Can you work these out from the model? Positions are in its coordinate system, mm. A direction names the side the tool comes from. Give positions to 0.01 mm unless a question says otherwise; leave off trailing zeros. Order: outer loops, then holes, each group sorted by start corner. A loop starts at its lowest first (then second) coordinate and runs counter-clockwise, first axis right, second up. Notation, with made-up numbers: (5.5, -32.5) -> (28.5, -32.5) arc R35 cw to (28.5, 3.5) -> close; hole circle Ø2 at (-11, 48). An arc over 180 degrees is marked (long way). Answer as CSV lines item,"result".
```python
from build123d import *

# Parameters (mm, degrees)
SKETCH1_R           = 2.1
BOSS_EXTRUDE1_DEPTH = 90
SKETCH5_R           = 2.5
CUT_EXTRUDE1_DEPTH  = 5
SKETCH6_R           = 8.4
SKETCH6_R_2         = 8
CUT_EXTRUDE2_DEPTH  = 4.2
FILLET1_START       = -1
FILLET1_DEPTH       = 5.2
CUT_EXTRUDE3_START  = -8
SKETCH7_R           = 8.4
SKETCH7_R_2         = 8
CUT_EXTRUDE3_DEPTH  = 8
SKETCH8_R           = 4.3
CUT_EXTRUDE4_DEPTH  = 4.2
FILLET2_START       = 82
FILLET2_DEPTH       = 9
SKETCH9_R           = 5
CUT_EXTRUDE5_DEPTH  = 85.8
SKETCH10_R          = 4.2
CUT_EXTRUDE6_DEPTH  = 4.2
BOSS_EXTRUDE2_START = 1.4
SKETCH11_W          = 90
SKETCH11_H          = 20
SKETCH11_R          = 2.5
BOSS_EXTRUDE2_DEPTH = 1.4


with BuildPart() as part:
    # Sketch1 → Boss-Extrude1 (new body)
    with BuildSketch(Plane.XY):
        with BuildLine():
            Line((8.4, 0), (31.8, 0))
            ThreePointArc((31.8, 0), (37.739696962, 2.460303038), (40.2, 8.4))
            Line((40.2, 8.4), (40.2, 31.8))
            ThreePointArc((40.2, 31.8), (37.739696962, 37.739696962), (31.8, 40.2))
            Line((31.8, 40.2), (8.4, 40.2))
            ThreePointArc((8.4, 40.2), (2.460303038, 37.739696962), (0, 31.8))
            Line((0, 31.8), (0, 8.4))
            ThreePointArc((0, 8.4), (2.460303038, 2.460303038), (8.4, 0))
        make_face()
        with Locations(Location((8.4, 31.8, 0), (0, 0, 180))):
            Circle(SKETCH1_R, mode=Mode.SUBTRACT)
        with Locations(Location((31.8, 31.8, 0), (0, 0, 180))):
            Circle(SKETCH1_R, mode=Mode.SUBTRACT)
        with Locations(Location((31.8, 8.4, 0), (0, 0, 180))):
            Circle(SKETCH1_R, mode=Mode.SUBTRACT)
        with Locations(Location((8.4, 8.4, 0), (0, 0, 180))):
            Circle(SKETCH1_R, mode=Mode.SUBTRACT)
    extrude(amount=BOSS_EXTRUDE1_DEPTH)

    # Sketch5 → Cut-Extrude1 (cut)
    with BuildSketch(Plane(origin=(40.2, 0, 0), x_dir=(0, 0, -1), z_dir=(1, 0, 0))):
        with Locations((-82, 20.1)):
            Circle(SKETCH5_R)
        with Locations((-8, 20.1)):
            Circle(SKETCH5_R)
    extrude(amount=-CUT_EXTRUDE1_DEPTH, mode=Mode.SUBTRACT)

    # Sketch6 → Cut-Extrude2 (cut)
    # profile 1 of 4: a face of its own
    with BuildSketch(Plane(origin=(0, 0, 0), x_dir=(-1, 0, 0), z_dir=(0, 0, -1))):
        with Locations((-31.8, 31.8)):
            Circle(SKETCH6_R)
        with Locations((-31.8, 31.8)):
            Circle(SKETCH6_R_2, mode=Mode.SUBTRACT)
    # profile 2 of 4: a face of its own
    with BuildSketch(Plane(origin=(0, 0, 0), x_dir=(-1, 0, 0), z_dir=(0, 0, -1))):
        with Locations((-8.4, 31.8)):
            Circle(SKETCH6_R)
        with Locations((-8.4, 31.8)):
            Circle(SKETCH6_R_2, mode=Mode.SUBTRACT)
    # profile 3 of 4: a face of its own
    with BuildSketch(Plane(origin=(0, 0, 0), x_dir=(-1, 0, 0), z_dir=(0, 0, -1))):
        with Locations((-8.4, 8.4)):
            Circle(SKETCH6_R)
        with Locations((-8.4, 8.4)):
            Circle(SKETCH6_R_2, mode=Mode.SUBTRACT)
    # profile 4 of 4: a face of its own
    with BuildSketch(Plane(origin=(0, 0, 0), x_dir=(-1, 0, 0), z_dir=(0, 0, -1))):
        with Locations((-31.8, 8.4)):
            Circle(SKETCH6_R)
        with Locations((-31.8, 8.4)):
            Circle(SKETCH6_R_2, mode=Mode.SUBTRACT)
    extrude(amount=-CUT_EXTRUDE2_DEPTH, mode=Mode.SUBTRACT)

    # Fillet1: read off the stored shape, not the designer's step
    # Fillet1 outline → Fillet1 (cut)
    with BuildSketch(Plane.XY.offset(FILLET1_START)):
        with BuildLine():
            ThreePointArc((0, 8.4), (0.024888944, 9.046153846), (0.099408284, 9.688478624))
            ThreePointArc((0.099408284, 9.688478624), (0.046153846, 9.646296288), (0, 9.69614814))
            Line((0, 9.69614814), (0, 8.4))
        make_face()
        with BuildLine():
            ThreePointArc((9.69614814, 0), (9.646296288, 0.046153846), (9.688478624, 0.099408284))
            ThreePointArc((9.688478624, 0.099408284), (9.046153846, 0.024888944), (8.4, 0))
            Line((8.4, 0), (9.69614814, 0))
        make_face()
        with BuildLine():
            Line((0, 31.8), (0, 30.50385186))
            ThreePointArc((0, 30.50385186), (0.046153846, 30.553703712), (0.099408284, 30.511521376))
            ThreePointArc((0.099408284, 30.511521376), (0.024888944, 31.153846154), (0, 31.8))
        make_face()
        with BuildLine():
            ThreePointArc((30.511521376, 0.099408284), (30.553703712, 0.046153846), (30.50385186, 0))
            Line((30.50385186, 0), (31.8, 0))
            ThreePointArc((31.8, 0), (31.153846154, 0.024888944), (30.511521376, 0.099408284))
        make_face()
        with BuildLine():
            ThreePointArc((8.4, 40.2), (9.046153846, 40.175111056), (9.688478624, 40.100591716))
            ThreePointArc((9.688478624, 40.100591716), (9.646296288, 40.153846154), (9.69614814, 40.2))
            Line((9.69614814, 40.2), (8.4, 40.2))
        make_face()
        with BuildLine():
            ThreePointArc((40.2, 9.69614814), (40.153846154, 9.646296288), (40.100591716, 9.688478624))
            ThreePointArc((40.100591716, 9.688478624), (40.175111056, 9.046153846), (40.2, 8.4))
            Line((40.2, 8.4), (40.2, 9.69614814))
        make_face()
        with BuildLine():
            Line((31.8, 40.2), (30.50385186, 40.2))
            ThreePointArc((30.50385186, 40.2), (30.553703712, 40.153846154), (30.511521376, 40.100591716))
            ThreePointArc((30.511521376, 40.100591716), (31.153846154, 40.175111056), (31.8, 40.2))
        make_face()
        with BuildLine():
            ThreePointArc((40.100591716, 30.511521376), (40.153846154, 30.553703712), (40.2, 30.50385186))
            Line((40.2, 30.50385186), (40.2, 31.8))
            ThreePointArc((40.2, 31.8), (40.175111056, 31.153846154), (40.100591716, 30.511521376))
        make_face()
    extrude(amount=FILLET1_DEPTH, mode=Mode.SUBTRACT)

    # Sketch7 → Cut-Extrude3 (cut)
    # profile 1 of 4: a face of its own
    with BuildSketch(Plane.XY.offset(90).offset(CUT_EXTRUDE3_START)):
        with Locations((8.4, 31.8)):
            Circle(SKETCH7_R)
        with Locations(Location((8.4, 31.8, 0), (0, 0, 180))):
            Circle(SKETCH7_R_2, mode=Mode.SUBTRACT)
    # profile 2 of 4: a face of its own
    with BuildSketch(Plane.XY.offset(90).offset(CUT_EXTRUDE3_START)):
        with Locations((31.8, 31.8)):
            Circle(SKETCH7_R)
        with Locations(Location((31.8, 31.8, 0), (0, 0, 180))):
            Circle(SKETCH7_R_2, mode=Mode.SUBTRACT)
    # profile 3 of 4: a face of its own
    with BuildSketch(Plane.XY.offset(90).offset(CUT_EXTRUDE3_START)):
        with Locations((31.8, 8.4)):
            Circle(SKETCH7_R)
        with Locations(Location((31.8, 8.4, 0), (0, 0, 180))):
            Circle(SKETCH7_R_2, mode=Mode.SUBTRACT)
    # profile 4 of 4: a face of its own
    with BuildSketch(Plane.XY.offset(90).offset(CUT_EXTRUDE3_START)):
        with Locations((8.4, 8.4)):
            Circle(SKETCH7_R)
        with Locations(Location((8.4, 8.4, 0), (0, 0, 180))):
            Circle(SKETCH7_R_2, mode=Mode.SUBTRACT)
    extrude(amount=CUT_EXTRUDE3_DEPTH, mode=Mode.SUBTRACT)

    # Sketch8 → Cut-Extrude4 (cut)
    with BuildSketch(Plane.XY.offset(90)):
        with Locations((8.4, 31.8)):
            Circle(SKETCH8_R)
        with Locations((31.8, 31.8)):
            Circle(SKETCH8_R)
        with Locations((31.8, 8.4)):
            Circle(SKETCH8_R)
        with Locations((8.4, 8.4)):
            Circle(SKETCH8_R)
    extrude(amount=-CUT_EXTRUDE4_DEPTH, mode=Mode.SUBTRACT)

    # Fillet2: read off the stored shape, not the designer's step
    # Fillet2 outline → Fillet2 (cut)
    with BuildSketch(Plane.XY.offset(FILLET2_START)):
        with BuildLine():
            ThreePointArc((0.099408284, 9.688478624), (0.046153846, 9.646296288), (0, 9.69614814))
            Line((0, 9.69614814), (0, 8.4))
            ThreePointArc((0, 8.4), (0.024888944, 9.046153846), (0.099408284, 9.688478624))
        make_face()
        with BuildLine():
            Line((0, 31.8), (0, 30.50385186))
            ThreePointArc((0, 30.50385186), (0.046153846, 30.553703712), (0.099408284, 30.511521376))
            ThreePointArc((0.099408284, 30.511521376), (0.024888944, 31.153846154), (0, 31.8))
        make_face()
        with BuildLine():
            ThreePointArc((9.69614814, 0), (9.646296288, 0.046153846), (9.688478624, 0.099408284))
            ThreePointArc((9.688478624, 0.099408284), (9.046153846, 0.024888944), (8.4, 0))
            Line((8.4, 0), (9.69614814, 0))
        make_face()
        with BuildLine():
            ThreePointArc((8.4, 40.2), (9.046153846, 40.175111056), (9.688478624, 40.100591716))
            ThreePointArc((9.688478624, 40.100591716), (9.646296288, 40.153846154), (9.69614814, 40.2))
            Line((9.69614814, 40.2), (8.4, 40.2))
        make_face()
        with BuildLine():
            ThreePointArc((30.511521376, 0.099408284), (30.553703712, 0.046153846), (30.50385186, 0))
            Line((30.50385186, 0), (31.8, 0))
            ThreePointArc((31.8, 0), (31.153846154, 0.024888944), (30.511521376, 0.099408284))
        make_face()
        with BuildLine():
            Line((31.8, 40.2), (30.50385186, 40.2))
            ThreePointArc((30.50385186, 40.2), (30.553703712, 40.153846154), (30.511521376, 40.100591716))
            ThreePointArc((30.511521376, 40.100591716), (31.153846154, 40.175111056), (31.8, 40.2))
        make_face()
        with BuildLine():
            ThreePointArc((40.2, 9.69614814), (40.153846154, 9.646296288), (40.100591716, 9.688478624))
            ThreePointArc((40.100591716, 9.688478624), (40.175111056, 9.046153846), (40.2, 8.4))
            Line((40.2, 8.4), (40.2, 9.69614814))
        make_face()
        with BuildLine():
            ThreePointArc((40.2, 31.8), (40.175111056, 31.153846154), (40.100591716, 30.511521376))
            ThreePointArc((40.100591716, 30.511521376), (40.153846154, 30.553703712), (40.2, 30.50385186))
            Line((40.2, 30.50385186), (40.2, 31.8))
        make_face()
    extrude(amount=FILLET2_DEPTH, mode=Mode.SUBTRACT)

    # Sketch9 → Cut-Extrude5 (cut)
    with BuildSketch(Plane.XY.offset(90)):
        with Locations((20.1, 20.1)):
            Circle(SKETCH9_R)
    extrude(amount=-CUT_EXTRUDE5_DEPTH, mode=Mode.SUBTRACT)

    # Sketch10 → Cut-Extrude6 (cut)
    with BuildSketch(Plane(origin=(0, 0, 0), x_dir=(-1, 0, 0), z_dir=(0, 0, -1))):
        with Locations((-31.8, 31.8)):
            Circle(SKETCH10_R)
        with Locations((-8.4, 31.8)):
            Circle(SKETCH10_R)
        with Locations((-31.8, 8.4)):
            Circle(SKETCH10_R)
        with Locations((-8.4, 8.4)):
            Circle(SKETCH10_R)
    extrude(amount=-CUT_EXTRUDE6_DEPTH, mode=Mode.SUBTRACT)

    # Sketch11 → Boss-Extrude2 (add)
    with BuildSketch(Plane(origin=(40.2, 0, 0), x_dir=(0, 0, -1), z_dir=(1, 0, 0)).offset(BOSS_EXTRUDE2_START)):
        with Locations((-45, 20.1)):
            Rectangle(SKETCH11_W, SKETCH11_H)
        with Locations((-82, 20.1)):
            Circle(SKETCH11_R, mode=Mode.SUBTRACT)
        with Locations((-8, 20.1)):
            Circle(SKETCH11_R, mode=Mode.SUBTRACT)
    extrude(amount=-BOSS_EXTRUDE2_DEPTH)


solid = part.part
```
Item 1: Please list where these lines run through material, in increasing order: line 1 along Y through (x, z) = (8.4, 87.3); line 2 along Z through (x, y) = (40, 20); line 3 along Y through (x, z) = (8.4, 1.95).
Numbers:
line 1,"y = 0.4 to 4.1, 12.7 to 16.4, 16.8 to 23.4, 23.8 to 27.5, 36.1 to 39.8"
line 2,"z = 0 to 5.5, 10.5 to 79.5, 84.5 to 90"
line 3,"y = 0.4 to 4.2, 12.6 to 16.4, 16.8 to 23.4, 23.8 to 27.6, 36 to 39.8"
Item 2: For pin 1 (4 mm diameter, centred on y = 20.1, z = 82, fed in from +X); pin 2 (6.5 mm diameter, centred on x = 31.8, y = 8.4, fed in from +Z); pin 3 (2.5 mm diameter, centred on x = 10, y = 31, fed in from -Z), each with a flat end and sliding along its axis, tell me the tip position at first contact or that it passes through.
Numbers:
pin 1,"stops at x = 35.2"
pin 2,"stops at z = 85.8"
pin 3,"stops at z = 4.2"
Item 3: Imagine slicing it at A-A, the plane z = 83. Give the number of separate pieces and of enclosed holes in the cut face, then the cut area to 3 significant figures.
Numbers:
separate pieces,"5"
enclosed holes,"5"
area,"1,340 mm²"
Item 4: For faces 5 (the flat face through (35, 28, 0)), 6 (the cylindrical face through (1.01, 11.46, 85.94)), 7 (the flat face through (40, 32, 4.2)), which set-ups out of +Z, -Z, +X, -X, +Y, -Y let a thin tool reach every point of the face, with its end or its side?
Numbers:
face 5,"-Z, +X, -X, +Y, -Y"
face 6,"+Z"
face 7,"-Z"
Item 5: We'd pull the mould along Z, two halves only. Please class faces 1 (the cylindrical face through (37.805, 37.674, 42.555)), 2 (the flat face through (11, 24, 4.2)), 3 (the flat face through (34, 9, 85.8)), 4 (the flat face through (35.2, 20, 8)): released by +Z, released by -Z, zero draft, split by the parting line, or undercut.
Numbers:
face 1,"zero draft"
face 2,"released by -Z"
face 3,"released by +Z"
face 4,"undercut"
Item 6: Imagine slicing it at D-D, the plane y = 20.1. Please give me the cut outline in (x, z).
Numbers:
outline,"(0, 0) -> (41.6, 0) -> (41.6, 5.5) -> (35.2, 5.5) -> (35.2, 10.5) -> (41.6, 10.5) -> (41.6, 79.5) -> (35.2, 79.5) -> (35.2, 84.5) -> (41.6, 84.5) -> (41.6, 90) -> (25.1, 90) -> (25.1, 4.2) -> (15.1, 4.2) -> (15.1, 90) -> (0, 90) -> close"
Item 7: Imagine slicing it at B-B, the plane z = 56.5. Please give me the cut outline in (x, y), then the cut area to 3 significant figures.
Numbers:
outline,"(0, 8.4) arc R8.4 ccw to (8.4, 0) -> (31.8, 0) arc R8.4 ccw to (40.2, 8.4) -> (40.2, 10.1) -> (41.6, 10.1) -> (41.6, 30.1) -> (40.2, 30.1) -> (40.2, 31.8) arc R8.4 ccw to (31.8, 40.2) -> (8.4, 40.2) arc R8.4 ccw to (0, 31.8) -> close; hole circle Ø4.2 at (8.4, 8.4); hole circle Ø4.2 at (8.4, 31.8); hole circle Ø10 at (20.1, 20.1); hole circle Ø4.2 at (31.8, 8.4); hole circle Ø4.2 at (31.8, 31.8)"
area,"1,450 mm²"
